For this review, take the finished solid that the model builds, in its own axes (mm). A direction names the side the tool comes from. Give positions to 0.01 mm unless a question says otherwise; leave off trailing zeros. Order: outer loops, then holes, each group sorted by start corner. A loop starts at its lowest first (then second) coordinate and runs counter-clockwise, first axis right, second up. Notation, with made-up numbers: (18, 60.5) - (59, 60.5) arc R23 ccw to (59, 89.5) - close; hole circle Ø4 at (-10.75, 77). An arc over 180 degrees is marked (long way). One line per item, written item: value.
```python
from build123d import *

# Parameters (mm, degrees)
SKETCH_R     = 1
SKETCH_R_2   = 2.5
PAD_DEPTH    = 2
SKETCH001_W  = 2
SKETCH001_H  = 2
POCKET_DEPTH = 2.001


with BuildPart() as part:
    # Sketch → Pad (new body)
    with BuildSketch(Plane.XY):
        with BuildLine():
            Line((-8.75, 3.5), (8.75, 3.5))
            ThreePointArc((4.167424, -3.5), (12.9333, -4.238613), (8.75, 3.5))
            Line((-4.167424, -3.5), (4.167424, -3.5))
            ThreePointArc((-8.75, 3.5), (-12.9333, -4.238613), (-4.167424, -3.5))
        make_face()
        Circle(SKETCH_R, mode=Mode.SUBTRACT)
        with Locations((-8.75, -1.5)):
            Circle(SKETCH_R_2, mode=Mode.SUBTRACT)
        with Locations((8.75, -1.5)):
            Circle(SKETCH_R_2, mode=Mode.SUBTRACT)
    extrude(amount=PAD_DEPTH)

    # Sketch001 → Pocket (cut, through all)
    with BuildSketch(Plane.XY.offset(2)):
        with Locations((-8.75, 0.5)):
            Rectangle(SKETCH001_W, SKETCH001_H)
        with Locations((8.75, 0.5)):
            Rectangle(SKETCH001_W, SKETCH001_H)
    extrude(amount=-POCKET_DEPTH, mode=Mode.SUBTRACT)


solid = part.part
```
(1) Take a section at A-A (y = -1.5). Write out the cut boundary in (x, z).
Answers below:
outline: (-13.75, 0) - (-11.25, 0) - (-11.25, 2) - (-13.75, 2) - close; (-6.25, 0) - (6.25, 0) - (6.25, 2) - (-6.25, 2) - close; (11.25, 0) - (13.75, 0) - (13.75, 2) - (11.25, 2) - close
(2) For P1, Ø0.6, axis at y = 1, z = 0.5, coming from the +X side; P2, Ø0.6, axis at x = -9, z = 1.5, coming from the -Y side; P3, Ø0.8, axis at y = 1, z = 1, coming from the -X side; P4, Ø0.6, axis at x = -1.5, z = 1, coming from the -Y side, all flat-tipped, find the tip position at first contact; note any pin that passes through.
Answers below:
P1: stops at x = 13.24
P2: stops at y = -6.5
P3: stops at x = -13.29
P4: stops at y = -3.5
(3) Take a section at B-B (x = 0). Write out the cut boundary in (y, z).
Answers below:
outline: (-3.5, 0) - (-1, 0) - (-1, 2) - (-3.5, 2) - close; (1, 0) - (3.5, 0) - (3.5, 2) - (1, 2) - close
(4) Draft analysis for pull direction X (two halves, no side actions). For faces 4 (the face through (0, -1, 1)), 5 (the face through (0, 3.5, 1)), state which applies: pulls with the +X half, pulls with the -X half, needs draft (parallel to the pull), parting line crosses it, or undercut.
Answers below:
face 4: undercut
face 5: needs draft
(5) Wall thickness on line 1 (X direction, y = -1.5, z = 0.7); line 2 (Y direction, x = -8.75, z = 1.25); line 3 (X direction, y = -0.5, z = 0.3): over which ranges is each line inside the solid? List them lowest first. Write a range as from..to.
Answers below:
line 1: x = -13.75..-11.25, -6.25..6.25, 11.25..13.75
line 2: y = -6.5..-4, 1.5..3.5
line 3: x = -13.65..-11.04, -6.46..-0.87, 0.87..6.46, 11.04..13.65
(6) Take a section at C-C (z = 0.85). Write out the cut boundary in (x, y), then the cut area to 3 significant figures.
Answers below:
outline: (-8.75, 3.5) arc R5 ccw (long way) to (-4.17, -3.5) - (4.17, -3.5) arc R5 ccw (long way) to (8.75, 3.5) - close; hole (-9.75, 0.79) arc R2.5 ccw (long way) to (-7.75, 0.79) - (-7.75, 1.5) - (-9.75, 1.5) - close; hole circle Ø2 at (0, 0); hole (7.75, 0.79) arc R2.5 ccw (long way) to (9.75, 0.79) - (9.75, 1.5) - (7.75, 1.5) - close
area: 176 mm^2
(7) Take a section at D-D (y = 0). Write out the cut boundary in (x, z), then the cut area to 3 significant figures.
Answers below:
outline: (-13.52, 0) - (-10.75, 0) - (-10.75, 2) - (-13.52, 2) - close; (-6.75, 0) - (-1, 0) - (-1, 2) - (-6.75, 2) - close; (1, 0) - (6.75, 0) - (6.75, 2) - (1, 2) - close; (10.75, 0) - (13.52, 0) - (13.52, 2) - (10.75, 2) - close
area: 34.1 mm^2
(8) Machinability: for faces 1 (the face through (9, 1.5, 1)), 2 (the face through (0.2, -1.4, 2)), 3 (the face through (0, -3.5, 1)), which of the approach directions +Z, -Z, +X, -X, +Y, -Y give a long, thin tool a straight path to every point of the face, cutting with its end or side? Answer none if there is none.
Answers below:
face 1: +Z, -Z
face 2: +Z, +X, -X, +Y, -Y
face 3: +Z, -Z, -Y
